Source: CAD feature listing. Evaluate the final solid. Frame: model axes, mm. Round coordinates to 2 decimals unless told otherwise and drop trailing zeros. Write each loop counter-clockwise with the first axis right and the second up, starting at its lowest first coordinate (ties: lowest second). Pieces come first, ordered by that corner, then holes. Notation, with made-up numbers: M -15,50 L 30,50 A31 ccw 30,87 Z; hole C 13,22.5 d3. An arc over 180 degrees is marked long. Put each result on its own line as item: value. Start each with the question number.
Autodesk Inventor part; units mm, degrees
ref_plane "YZ Plane" through (0, 0, 0) normal (1, 0, 0) x (0, 1, 0)
ref_plane "XZ Plane" through (0, 0, 0) normal (0, 1, 0) x (-1, 0, 0)
ref_plane "XY Plane" through (0, 0, 0) normal (0, 0, 1) x (1, 0, 0)
sketch "Schizzo1" plane through (0, 0, 0) normal (0, 1, 0) x (-1, 0, 0)
  line L0 (20, 0) -> (65, 0)
  line L1 (85, -20) -> (85, -74)
  line L2 (65, -94) -> (20, -94)
  line L3 (0, -74) -> (0, -20)
  arc A0 (85, -20) -> (65, 0) centre (65, -20) ccw
  arc A1 (20, 0) -> (0, -20) centre (20, -20) ccw
  arc A2 (0, -74) -> (20, -94) centre (20, -74) ccw
  arc A3 (65, -94) -> (85, -74) centre (65, -74) ccw
  circle A4 centre (74, -7) radius 1.75
  circle A5 centre (74, -87) radius 1.75
  circle A6 centre (11, -87) radius 1.75
  circle A7 centre (11, -7) radius 1.75
  circle A8 centre (46.5, -41.3) radius 0.5
  circle A9 centre (46.5, -43.2) radius 0.5
  circle A10 centre (46.5, -45.1) radius 0.5
  circle A11 centre (46.5, -47) radius 0.5
  circle A12 centre (46.5, -48.9) radius 0.5
  circle A13 centre (46.5, -50.8) radius 0.5
  circle A14 centre (46.5, -52.7) radius 0.5
  circle A15 centre (44.6, -41.3) radius 0.5
  circle A16 centre (44.6, -43.2) radius 0.5
  circle A17 centre (44.6, -45.1) radius 0.5
  circle A18 centre (44.6, -47) radius 0.5
  circle A19 centre (44.6, -48.9) radius 0.5
  circle A20 centre (44.6, -50.8) radius 0.5
  circle A21 centre (44.6, -52.7) radius 0.5
  circle A22 centre (42.7, -41.3) radius 0.5
  circle A23 centre (42.7, -43.2) radius 0.5
  circle A24 centre (42.7, -45.1) radius 0.5
  circle A25 centre (42.7, -47) radius 0.5
  circle A26 centre (42.7, -48.9) radius 0.5
  circle A27 centre (42.7, -50.8) radius 0.5
  circle A28 centre (42.7, -52.7) radius 0.5
  circle A29 centre (40.8, -41.3) radius 0.5
  circle A30 centre (40.8, -43.2) radius 0.5
  circle A31 centre (40.8, -45.1) radius 0.5
  circle A32 centre (40.8, -47) radius 0.5
  circle A33 centre (40.8, -48.9) radius 0.5
  circle A34 centre (40.8, -50.8) radius 0.5
  circle A35 centre (40.8, -52.7) radius 0.5
  point P0 (46.5, -48.9)
  point P1 (46.5, -48.9)
  point P2 (44.6, -48.9)
  point P3 (42.7, -48.9)
  point P4 (40.8, -48.9)
  dimension "d20" = 3.5
  dimension "d21" = 3.5
  dimension "d22" = 3.5
  dimension "d23" = 3.5
  dimension "d29" = 1.9
  dimension "d32" = 1.9
  dimension "d37" = 1.9
  dimension "d40" = 1.9
  dimension "d43" = 1
  dimension "d46" = 1.9
  dimension "d49" = 1.9
extrude "Estrusione1" add sketch "Schizzo1" along normal blind 1.8
properties part number "pcb"
(1) Pull-direction query (Z, two-part tool) for faces 1 (the cylindrical face through (-5.703, 0.887, -6.014)), 2 (the cylindrical face through (-11.81, 0.89, -5.45)), 3 (the cylindrical face through (-6.014, 0.887, -88.297)), 4 (the flat face through (-42, 1.8, -46)); classes: +Z half, -Z half, draft (parallel to the pull), parting line (faces both ways), or undercut.
(2) Section query C-C (z = -83.5). Return loops of the section in (x, y).
(3) Section query B-B (x = -6.5). Return loops of the section in (y, z), and give its area (3 significant figures).
(4) Section query A-A (y = 0.7). Count the separate pieces of the cut face and the enclosed holes in it, and give its area (3 significant figures).
(5) Ray query, line 1 along X through (y, z) = (1.05, -52.7); line 2 along Z through (x, y) = (-74, 0.6); line 3 along Z through (x, y) = (-19.5, 0.9). Return the intervals inside material, ascending.
(6) Contact query for a flat-ended pin moving along its axis: P1, Ø2, axis at x = -74, z = -87, coming from the -Y side. Output: stop coordinate, or through.
Entries:
1. face 1: +Z half
1. face 2: undercut
1. face 3: -Z half
1. face 4: draft
2. outline: M -82.6,0 L -2.4,0 L -2.4,1.8 L -82.6,1.8 Z
3. outline: M 0,-88.76 L 1.8,-88.76 L 1.8,-5.24 L 0,-5.24 Z
3. area: 150 mm2
4. separate pieces: 1
4. enclosed holes: 32
4. area: 7,590 mm2
5. line 1: -85 to -47, -46 to -45.1, -44.1 to -43.2, -42.2 to -41.3, -40.3 to 0
5. line 2: -91.86 to -88.75, -85.25 to -8.75, -5.25 to -2.14
5. line 3: -93.99 to -0.01
6. P1: through
